```python
from build123d import *

# Parameters (mm, degrees)
F0_W      = 35
F0_H      = 35
F1_DEPTH  = 4
F2_R      = 3
F2_R_2    = 1.675
F4_DEPTH  = 2
F5_R      = 5
F6_DEPTH  = 12.5
F3_W      = 35
F3_H      = 6
F7_DEPTH  = 35
F8_R      = 6
F8_R_2    = 1.5
F9_DEPTH  = 6.001
F11_D     = 5
F11_DEPTH = 2
F11_TIP   = 1.5021515476


with BuildPart() as f1:
    # F0 (on Top) → F1 (new body)
    with BuildSketch(Plane.XY):
        with Locations((17.5, 17.5)):
            Rectangle(F0_W, F0_H)
    extrude(amount=F1_DEPTH)

    # F2 (on face) → F4 (cut)
    with BuildSketch(Plane.XY.offset(4)):
        with BuildLine():
            ThreePointArc((13, 21), (10, 24), (7, 21))
            ThreePointArc((7, 21), (10, 18), (13, 21))
        make_face()
        with BuildLine():
            ThreePointArc((8.325, 21), (10, 22.675), (11.675, 21))
            ThreePointArc((11.675, 21), (10, 19.325), (8.325, 21))
        make_face(mode=Mode.SUBTRACT)
        with Locations((25, 21)):
            Circle(F2_R)
        with Locations((25, 21)):
            Circle(F2_R_2, mode=Mode.SUBTRACT)
        with Locations((25, 6)):
            Circle(F2_R)
        with Locations((25, 6)):
            Circle(F2_R_2, mode=Mode.SUBTRACT)
        with BuildLine():
            ThreePointArc((13, 6), (7.8786796564, 8.1213203436), (10, 3))
            ThreePointArc((10, 3), (12.1213203436, 3.8786796564), (13, 6))
        make_face()
        with BuildLine():
            ThreePointArc((11.675, 6), (11.1844038585, 4.8155961415), (10, 4.325))
            ThreePointArc((10, 4.325), (8.8155961415, 7.1844038585), (11.675, 6))
        make_face(mode=Mode.SUBTRACT)
    extrude(amount=-F4_DEPTH, mode=Mode.SUBTRACT)

    # F5
    f5_edges = [f1.edges().sort_by_distance(p)[0] for p in [
        (0, 0, 2),
        (35, 0, 2),
    ]]
    fillet(f5_edges, radius=F5_R)

    # F2 (on face) → F6 (cut, symmetric)
    with BuildSketch(Plane.XY.offset(4)):
        with BuildLine():
            ThreePointArc((8.325, 21), (10, 19.325), (11.675, 21))
            ThreePointArc((11.675, 21), (10, 22.675), (8.325, 21))
        make_face()
        with Locations((25, 21)):
            Circle(F2_R_2)
        with Locations((25, 6)):
            Circle(F2_R_2)
        with BuildLine():
            ThreePointArc((11.675, 6), (8.8155961415, 7.1844038585), (10, 4.325))
            ThreePointArc((10, 4.325), (11.1844038585, 4.8155961415), (11.675, 6))
        make_face()
    extrude(amount=F6_DEPTH, both=True, mode=Mode.SUBTRACT)

    # F3 (on face) → F7 (join)
    with BuildSketch(Plane.XY.offset(4)):
        with Locations((17.5, 32)):
            Rectangle(F3_W, F3_H)
    extrude(amount=F7_DEPTH)

    # F8 (on face) → F9 (cut, through all)
    with BuildSketch(Plane.XZ.offset(-29)):
        with Locations((17.5, 20.5)):
            Circle(F8_R)
        with Locations((30, 33)):
            Circle(F8_R_2)
        with Locations((5, 33)):
            Circle(F8_R_2)
        with Locations((5, 8)):
            Circle(F8_R_2)
        with Locations((30, 8)):
            Circle(F8_R_2)
    extrude(amount=-F9_DEPTH, mode=Mode.SUBTRACT)

    # F11
    with Locations(Plane(origin=(0, 35, 0), x_dir=(-1, 0, 0), z_dir=(0, 1, 0))):
        with Locations((-30, 33), (-30, 8), (-5, 8), (-5, 33)):
            Hole(F11_D / 2, depth=F11_DEPTH)
            with Locations((0, 0, -(F11_DEPTH + F11_TIP / 2))):  # 118° drill point
                Cone(0, F11_D / 2, F11_TIP, mode=Mode.SUBTRACT)


solid = f1.part
```
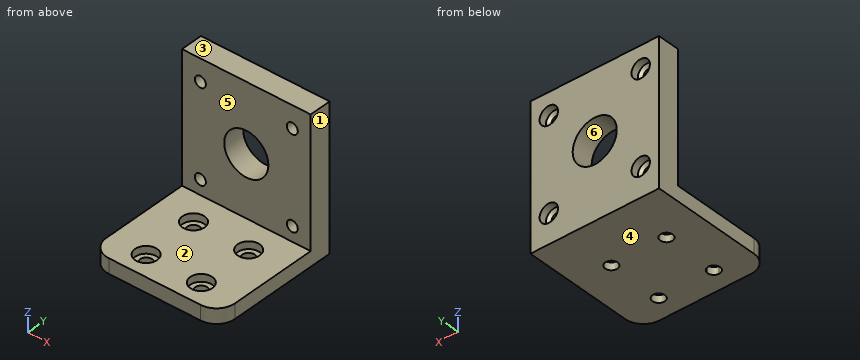
CAD build for the part. Positions are in the model's coordinates, mm. Face numbers are marked on the shaded views. A direction names the side the tool comes from. Round coordinates to 2 decimals unless told otherwise and drop trailing zeros. Loops run counter-clockwise (first coordinate to the right, second up) from the corner with the lowest first, then second, coordinate; pieces in that order, holes last. Notation, with made-up numbers: M -7.75,42 L 18.25,42 A14 cw 18.25,68 Z; hole C 49.5,-3 d7. An arc over 180 degrees is marked long. Use a Markdown table: item, result. Add a question column.
(1) Which spindle directions (+Z, -Z, +X, -X, +Y, -Y) get a long thin tool onto all of the face, cutting with end or side? Do the marked faces 1 and 2. Say none if no direction does.
(2) Cut at C-C (x = 25). Give the cut face in (y, z) (3 decimals), and give its area (3 significant figures).
(3) Pull direction Z, two halves, no side cores. Call the marked faces 3, 4, 5 and 6: +Z half, -Z half, draft (parallel to the pull), parting line (faces both ways), or undercut.
(4) Drill centre lines: line 1 (X direction, y = 29.5, z = 33); line 2 (Y direction, x = 10, z = 0.5) (3 decimals); line 3 (Z direction, x = 5, y = 33.6). Where is each one in solid material? Low to high.
(5) Cut at A-A (x = 17.5). Give the cut face in (y, z).
(6) Cut at B-B (z = 33). Give the cut face in (x, y), and give its area (3 significant figures).
(7) Cut at D-D (y = 31). Give the cut face in (x, z).
(8) Flat gauge pins, fed straight in: pin 1 (5 mm diameter, centred on x = 25, y = 6, fed in from +Z); pin 2 (12 mm diameter, centred on x = 22.5, y = 10, fed in from +Z); pin 3 (1.5 mm diameter, centred on x = 20.5, z = 17, fed in from -Y); pin 4 (8 mm diameter, centred on x = 5, z = 33, fed in from -Y). Where does each tip first touch, or does it go through?
Geometry says:
| question | item | result |
|---|---|---|
| 1 | face 1 | +Z, -Z, +X, +Y, -Y |
| 1 | face 2 | +Z, +X, -X, -Y |
| 2 | outline | M 0,0 L 4.325,0 L 4.325,2 L 3,2 L 3,4 L 0,4 Z; M 7.675,0 L 19.325,0 L 19.325,2 L 18,2 L 18,4 L 9,4 L 9,2 L 7.675,2 Z; M 22.675,0 L 35,0 L 35,39 L 29,39 L 29,4 L 24,4 L 24,2 L 22.675,2 Z |
| 2 | area | 313 mm² |
| 3 | face 3 | +Z half |
| 3 | face 4 | -Z half |
| 3 | face 5 | draft |
| 3 | face 6 | undercut |
| 4 | line 1 | x = 0 to 3.5, 6.5 to 28.5, 31.5 to 35 |
| 4 | line 2 | y = 0 to 4.325, 7.675 to 19.325, 22.675 to 35 |
| 4 | line 3 | z = 0 to 5.5, 10.5 to 30.5, 35.5 to 39 |
| 5 | outline | M 0,0 L 35,0 L 35,14.5 L 29,14.5 L 29,4 L 0,4 Z; M 29,26.5 L 35,26.5 L 35,39 L 29,39 Z |
| 6 | outline | M 0,29 L 3.5,29 L 3.5,32.4 L 2.5,33 L 2.5,35 L 0,35 Z; M 6.5,29 L 28.5,29 L 28.5,32.4 L 27.5,33 L 27.5,35 L 7.5,35 L 7.5,33 L 6.5,32.4 Z; M 31.5,29 L 35,29 L 35,35 L 32.5,35 L 32.5,33 L 31.5,32.4 Z |
| 6 | area | 165 mm² |
| 7 | outline | M 0,0 L 35,0 L 35,39 L 0,39 Z; hole C 5,8 d3; hole C 5,33 d3; hole C 17.5,20.5 d12; hole C 30,8 d3; hole C 30,33 d3 |
| 8 | pin 1 | stops at z = 2 |
| 8 | pin 2 | stops at z = 4 |
| 8 | pin 3 | passes through |
| 8 | pin 4 | stops at y = 29 |
